from build123d import *

# Parameters (mm, degrees)
BOSS_EXTRUDE1_DEPTH      = 65
BOSS_EXTRUDE1_DEPTH_BACK = 65
BOSS_EXTRUDE2_DEPTH      = 15


with BuildPart() as part:
    # Sketch1 → Boss-Extrude1 (new body, two sides)
    with BuildSketch(Plane(origin=(0, 0, 0), x_dir=(0, 0, -1), z_dir=(1, 0, 0))) as boss_extrude1_sk:
        with BuildLine():
            Line((-11, 11.5), (11, 11.5))
            ThreePointArc((11, 11.5), (22.5, 0), (11, -11.5))
            Line((11, -11.5), (-11, -11.5))
            ThreePointArc((-11, -11.5), (-22.5, 0), (-11, 11.5))
        make_face()
    extrude(amount=BOSS_EXTRUDE1_DEPTH)
    extrude(boss_extrude1_sk.sketch, amount=-BOSS_EXTRUDE1_DEPTH_BACK)

    # Sketch2 → Boss-Extrude2 (add)
    with BuildSketch(Plane.ZY.offset(65)):
        with BuildLine():
            Line((-2, 2), (2, 2))
            ThreePointArc((2, 2), (4, 0), (2, -2))
            Line((2, -2), (-2, -2))
            ThreePointArc((-2, -2), (-4, 0), (-2, 2))
        make_face()
    extrude(amount=BOSS_EXTRUDE2_DEPTH)


solid = part.part
Model file for the job. Use its own axes, mm. A direction names the side the tool comes from. Give positions to 0.01 mm unless a question says otherwise; leave off trailing zeros. Write each loop counter-clockwise with the first axis right and the second up, starting at its lowest first coordinate (ties: lowest second). Pieces come first, ordered by that corner, then holes. Notation, with made-up numbers: (23, 87.5) -> (60, 87.5) arc R29 cw to (60, 110.5) -> close; hole circle Ø11 at (-3, -38.75). An arc over 180 degrees is marked (long way). Write item = value, one per line.
(1) Slice it at C-C, the plane x = -49.5. Give the cut face in (y, z).
Determined:
outline = (-11.5, -11) arc R11.5 ccw to (11.5, -11) -> (11.5, 11) arc R11.5 ccw to (-11.5, 11) -> close
(2) Tool access for faces 1 (the face through (-72, -2, 0)), 2 (the face through (0.91, 0.253, -22.497)), 3 (the face through (-72, 0, 4)), 4 (the face through (-72, 2, 0)), 5 (the face through (-72, 0, -4)): list every direction of +Z, -Z, +X, -X, +Y, -Y with a clear straight run to the whole face (end or side of a thin tool).
Determined:
face_1 = +Z, -Z, -X, -Y
face_2 = -Z, +X, -X
face_3 = +Z, -X
face_4 = +Z, -Z, -X, +Y
face_5 = -Z, -X
(3) Slice it at A-A, the plane y = 0. Give the cut face in (x, z).
Determined:
outline = (-80, -4) -> (-65, -4) -> (-65, -22.5) -> (65, -22.5) -> (65, 22.5) -> (-65, 22.5) -> (-65, 4) -> (-80, 4) -> close
(4) Probe line 1 along X through (y, z) = (10.75, -3); line 2 along Z through (x, y) = (52.5, 0.75); line 3 along Y through (x, z) = (-72, -1). List the from-to ranges inside material, lowest first.
Determined:
line_1 = -65 to 65
line_2 = -22.48 to 22.48
line_3 = -2 to 2
(5) Slice it at B-B, the plane z = 7. Give the cut face in (x, y).
Determined:
outline = (-65, -11.5) -> (65, -11.5) -> (65, 11.5) -> (-65, 11.5) -> close
(6) Flat gauge pins, fed straight in: P1, Ø1.2, axis at x = -73.5, z = 1, coming from the -Y side; P2, Ø2, axis at x = -37, y = -8.5, coming from the +Z side; P3, Ø10, axis at x = -24, y = -9, coming from the -Z side. Where does each tip first touch, or does it go through?
Determined:
P1 = -2
P2 = 19.72
P3 = -21.78
